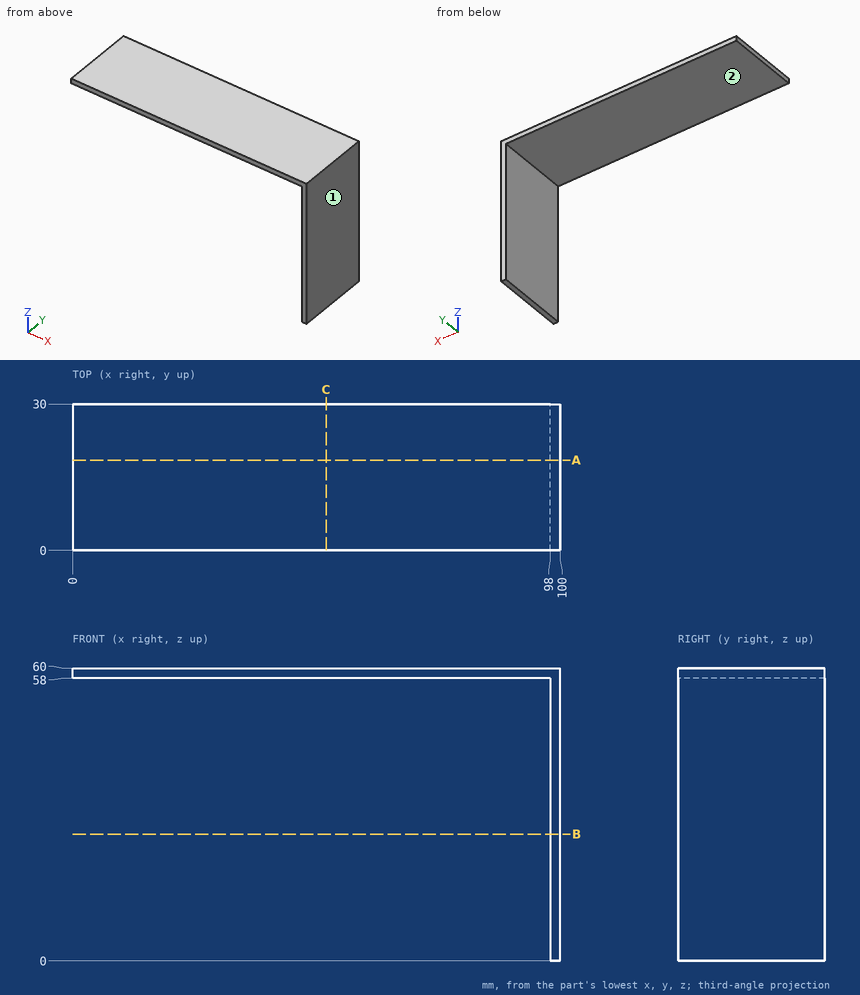
Job drawing, mm, ordinate dimensions from the low corner. One solid piece. A direction names the side the tool comes from. Coordinates: 2 decimals unless noted, no trailing zeros. Write each loop counter-clockwise with the first axis right and the second up, starting at its lowest first coordinate (ties: lowest second). Pieces come first, ordered by that corner, then holes.
Item 1: Probe line 1 (Z direction, x = 90, y = 27.75); line 2 (X direction, y = 8, z = 42). List the from-to ranges inside material, lowest first.
Item 2: Slice it at B-B (z = 26). Write the cut outline in (x, y).
Item 3: Slice it at A-A (y = 18.5). Write the cut outline in (x, z), and give its area (3 significant figures).
Item 4: Pin check, flat tips, straight feed: pin 1 (4 mm diameter, centred on y = 13.5, z = 25, fed in from -X); pin 2 (9 mm diameter, centred on x = 53, y = 13, fed in from -Z). Stop position of each tip, or through.
Item 5: Slice it at C-C (x = 52). Write the cut outline in (y, z).
Item 6: Which spindle directions (+Z, -Z, +X, -X, +Y, -Y) get a long thin tool onto all of the face, cutting with end or side? Do the marked faces 1 and 2. Say none if no direction does.
Results found:
1. line 1: z = 58 to 60
1. line 2: x = 98 to 100
2. outline: (98, 0) - (100, 0) - (100, 30) - (98, 30) - close
3. outline: (0, 58) - (98, 58) - (98, 0) - (100, 0) - (100, 60) - (0, 60) - close
3. area: 316 mm2
4. pin 1: stops at x = 98
4. pin 2: stops at z = 58
5. outline: (0, 58) - (30, 58) - (30, 60) - (0, 60) - close
6. face 1: +Z, -Z, +X, +Y, -Y
6. face 2: -Z, -X, +Y, -Y
